from build123d import *

# Parameters (mm, degrees)
SKETCH1_R           = 3.5
SKETCH1_R_2         = 2.5
BOSS_EXTRUDE1_DEPTH = 2.8
SKETCH2_R           = 3.5
SKETCH2_R_2         = 1.25
BOSS_EXTRUDE2_DEPTH = 0.2
SKETCH3_R           = 3.5
SKETCH3_R_2         = 2.5
BOSS_EXTRUDE3_DEPTH = 1
BOSS_EXTRUDE4_START = -1.5
BOSS_EXTRUDE4_DEPTH = 1.5


with BuildPart() as part:
    # Sketch1 → Boss-Extrude1 (new body)
    with BuildSketch(Plane.XY):
        Circle(SKETCH1_R)
        Circle(SKETCH1_R_2, mode=Mode.SUBTRACT)
    extrude(amount=BOSS_EXTRUDE1_DEPTH)

    # Sketch2 → Boss-Extrude2 (add)
    with BuildSketch(Plane.XY.offset(2.8)):
        Circle(SKETCH2_R)
        Circle(SKETCH2_R_2, mode=Mode.SUBTRACT)
    extrude(amount=BOSS_EXTRUDE2_DEPTH)

    # Sketch3 → Boss-Extrude3 (add)
    with BuildSketch(Plane.XY.offset(3)):
        Circle(SKETCH3_R)
        Circle(SKETCH3_R_2, mode=Mode.SUBTRACT)
    extrude(amount=BOSS_EXTRUDE3_DEPTH)

    # Sketch4 → Boss-Extrude4 (add)
    with BuildSketch(Plane.XY.offset(4).offset(BOSS_EXTRUDE4_START)):
        with BuildLine():
            Line((-3, -1.802775638), (-1.993399861, -14.162348377))
            ThreePointArc((-1.993399861, -14.162348377), (0, -16), (1.993399861, -14.162348377))
            Line((1.993399861, -14.162348377), (3, -1.802775638))
            ThreePointArc((3, -1.802775638), (0, -3.5), (-3, -1.802775638))
        make_face()
    extrude(amount=BOSS_EXTRUDE4_DEPTH)


solid = part.part
Could you check a few things on this model? Use its own coordinates, in mm. A direction names the side the tool comes from. Give positions to 0.01 mm unless a question says otherwise; leave off trailing zeros. Order: outer loops, then holes, each group sorted by start corner. A loop starts at its lowest first (then second) coordinate and runs counter-clockwise, first axis right, second up. Notation, with made-up numbers: (11, -32.75) -> (31, -32.75) arc R34 cw to (31, -0.75) -> close; hole circle Ø5 at (30, 77.25). An arc over 180 degrees is marked (long way). Return JSON: item names as keys, results as strings.
1. I need wall thicknesses on line 1 (Y direction, x = 0, z = 1.9); line 2 (Y direction, x = 0, z = 3.6); line 3 (Z direction, x = 0, y = -8.5). Which ranges of each line are inside material? Lowest first, please. Write a range as from..to.
Answer list:
{"line 1": "y = -3.5..-2.5, 2.5..3.5", "line 2": "y = -16..-2.5, 2.5..3.5", "line 3": "z = 2.5..4"}
2. Imagine slicing it at B-B on x = -0.75. List the corners of the cut face in (y, z) for me.
Answer list:
{"outline": "(-15.85, 2.5) -> (-3.42, 2.5) -> (-3.42, 0) -> (-2.38, 0) -> (-2.38, 2.8) -> (-1, 2.8) -> (-1, 3) -> (-2.38, 3) -> (-2.38, 4) -> (-15.85, 4) -> close; (1, 2.8) -> (2.38, 2.8) -> (2.38, 0) -> (3.42, 0) -> (3.42, 4) -> (2.38, 4) -> (2.38, 3) -> (1, 3) -> close"}
3. Thinking about a two-plate mould opening in X: for faces 4 (the cylindrical face through (0, -16, 3)), 5 (the flat face through (-2.504, -7.896, 3.24)), 6 (the flat face through (1, 1, 2.8)), which applies, pulls with the +X half, pulls with the -X half, needs draft (parallel to the pull), parting line crosses it, or undercut?
Answer list:
{"face 4": "parting line crosses it", "face 5": "pulls with the -X half", "face 6": "undercut"}
4. Imagine slicing it at D-D on x = 0. List the corners of the cut face in (y, z) for me, then the cut area to 4 significant figures.
Answer list:
{"outline": "(-16, 2.5) -> (-3.5, 2.5) -> (-3.5, 0) -> (-2.5, 0) -> (-2.5, 2.8) -> (-1.25, 2.8) -> (-1.25, 3) -> (-2.5, 3) -> (-2.5, 4) -> (-16, 4) -> close; (1.25, 2.8) -> (2.5, 2.8) -> (2.5, 0) -> (3.5, 0) -> (3.5, 4) -> (2.5, 4) -> (2.5, 3) -> (1.25, 3) -> close", "area": "27.25 mm2"}
5. Imagine slicing it at C-C on z = 1.85. List the corners of the cut face in (x, y) for me, then the cut area to 3 significant figures.
Answer list:
{"outline": "circle Ø7 at (0, 0); hole circle Ø5 at (0, 0)", "area": "18.8 mm2"}
6. On a 3-axis mill with a long thin cutter (end or side, diameter ignored), from which of +Z, -Z, +X, -X, +Y, -Y can I reach the whole of each face in a straight line? I mean faces 1 (the cylindrical face through (-0.54, -2.44, 1.38)), 2 (the cylindrical face through (-0.54, -2.44, 3.49)), 3 (the flat face through (2.49, -8.07, 3.24)). Say none if no direction works.
Answer list:
{"face 1": "-Z", "face 2": "+Z", "face 3": "+Z, -Z, +X, -Y"}
7. For pin 1 Ø3 at (x, y) = (0, 0) entering from +Z; pin 2 Ø1 at (x, y) = (0.5, -6.5) entering from -Z; pin 3 Ø1.5 at (x, z) = (0.5, 1.5) entering from -Y, each with a flat end and sliding along its axis, tell me the tip position at first contact or that it passes through.
Answer list:
{"pin 1": "stops at z = 3", "pin 2": "stops at z = 2.5", "pin 3": "stops at y = -3.5"}
8. Imagine slicing it at A-A on y = 0. List the corners of the cut face in (x, z) for me.
Answer list:
{"outline": "(-3.5, 0) -> (-2.5, 0) -> (-2.5, 2.8) -> (-1.25, 2.8) -> (-1.25, 3) -> (-2.5, 3) -> (-2.5, 4) -> (-3.5, 4) -> close; (1.25, 2.8) -> (2.5, 2.8) -> (2.5, 0) -> (3.5, 0) -> (3.5, 4) -> (2.5, 4) -> (2.5, 3) -> (1.25, 3) -> close"}
